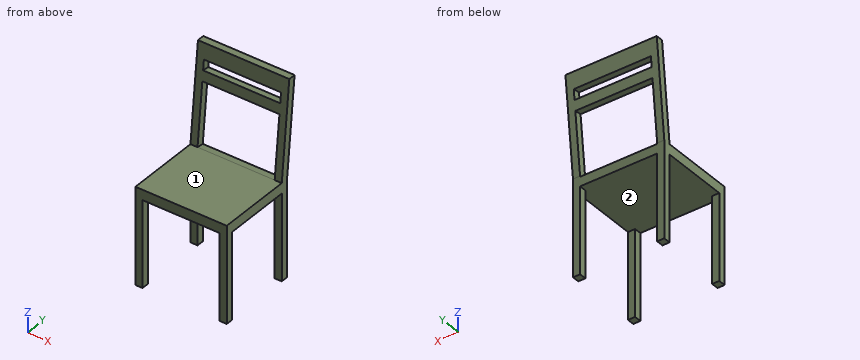
from build123d import *

# Parameters (mm, degrees)
F0_W     = 450
F0_H     = 450
F1_DEPTH = 950
F2_W     = 330
F2_H     = 425
F2_W_2   = 50
F2_H_2   = 50
F3_DEPTH = 450.001
F4_W     = 380
F4_H     = 425
F5_DEPTH = 450.001
F6_W     = 380
F6_H     = 302.6243293636
F6_H_2   = 50
F7_DEPTH = 134.2592361444


with BuildPart() as f1:
    # F0 (on Top) → F1 (new body)
    with BuildSketch(Plane.XY):
        Rectangle(F0_W, F0_H)
    extrude(amount=F1_DEPTH)

    # F2 (on face) → F3 (cut, through all)
    with BuildSketch(Plane.YZ.offset(225)):
        Polygon((-225, 475), (140, 475), (190, 950), (-225, 950), align=None)
        with Locations((-25, 212.5)):
            Rectangle(F2_W, F2_H)
        with Locations((200, 212.5)):
            Rectangle(F2_W_2, F2_H)
        with Locations((200, 450)):
            Rectangle(F2_W_2, F2_H_2)
        Polygon((175, 475), (225, 475), (225, 950), align=None)
    extrude(amount=-F3_DEPTH, mode=Mode.SUBTRACT)

    # F4 (on face) → F5 (cut, through all)
    with BuildSketch(Plane.XZ.offset(225)):
        with Locations((0, 212.5)):
            Rectangle(F4_W, F4_H)
    extrude(amount=-F5_DEPTH, mode=Mode.SUBTRACT)

    # F6 (on face) → F7 (cut, through all)
    with BuildSketch(Plane(origin=(0, 89.0136986301, -9.3698630137), x_dir=(1, 0, 0), z_dir=(0, -0.9945054529, 0.1046847845))):
        with Locations((0, 638.358124652)):
            Rectangle(F6_W, F6_H)
        with Locations((0, 864.6702893338)):
            Rectangle(F6_W, F6_H_2)
    extrude(amount=-F7_DEPTH, mode=Mode.SUBTRACT)


solid = f1.part
CAD build for the part. Positions are in the model's coordinates, mm. Face numbers are marked on the shaded views. Coordinates: 2 decimals unless noted, no trailing zeros. Loops run counter-clockwise (first coordinate to the right, second up) from the corner with the lowest first, then second, coordinate; pieces in that order, holes last. Notation, with made-up numbers: (47.5, 86) - (83.5, 86) arc R17 cw to (83.5, 93) - close; hole circle Ø7 at (-19.75, 54). An arc over 180 degrees is marked (long way). Use one line per item in the form item = value. Start each with the question number.
1) Band-saw the part on D-D (y = -66.5). Give the cut face in (x, z), and give its area (3 significant figures).
2) Band-saw the part on A-A (z = 93). Give the cut face in (x, y).
3) Drill centre lines: L1, parallel to X at y = 152.5, z = 422; L2, parallel to Z at x = 29.5, y = 105; L3, parallel to Y at x = 206, z = 725. Where is each one in solid material? Low to high. Write a range as from..to.
4) Two-plate mould, pull along X, no slides. Class the marked faces 1 and 2: +X half, -X half, draft (parallel to the pull), parting line (faces both ways), or undercut.
5) Band-saw the part on B-B (x = -27). Give the cut face in (y, z).
6) Band-saw the part on C-C (z = 846). Give the cut face in (x, y).
7) Flat gauge pins, fed straight in: pin 1 (6 mm diameter, centred on x = 153.5, y = 98, fed in from -Z); pin 2 (17.5 mm diameter, centred on x = 204, z = 146, fed in from +Y); pin 3 (12 mm diameter, centred on x = 38.5, y = -35.5, fed in from +Z). Where does each tip first touch, or does it go through?
Check values:
q1.outline = (-225, 425) - (225, 425) - (225, 475) - (-225, 475) - close
q1.area = 22,500 mm2
q2.outline = (-225, -225) - (-190, -225) - (-190, -190) - (-225, -190) - close; (-225, 140) - (-190, 140) - (-190, 175) - (-225, 175) - close; (190, -225) - (225, -225) - (225, -190) - (190, -190) - close; (190, 140) - (225, 140) - (225, 175) - (190, 175) - close
q3.L1 = -225..-190, 190..225
q3.L2 = 425..475
q3.L3 = 166.32..201.32
q4.face_1 = draft
q4.face_2 = undercut
q5.outline = (-225, 425) - (175, 425) - (175, 471.32) - (140, 475) - (-225, 475) - close; (171.68, 775.96) - (206.3, 772.32) - (211.53, 822.04) - (176.91, 825.69) - close; (182.15, 875.41) - (216.77, 871.77) - (225, 950) - (190, 950) - close
q6.outline = (-225, 179.05) - (-190, 179.05) - (-190, 214.05) - (-225, 214.05) - close; (190, 179.05) - (225, 179.05) - (225, 214.05) - (190, 214.05) - close
q7.pin_1 = 425
q7.pin_2 = 175
q7.pin_3 = 475
